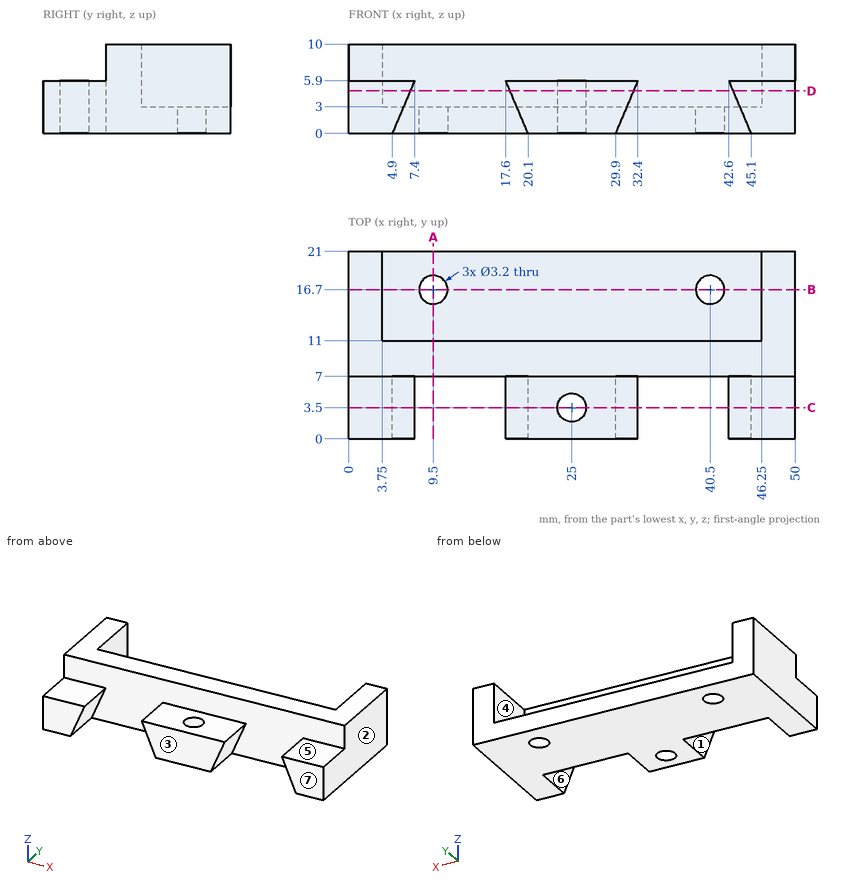
Print and shaded views of the part. All mm, measured from the part's lowest x, y and z. A direction names the side the tool comes from. Give positions to 0.01 mm unless a question says otherwise; leave off trailing zeros. Loops run counter-clockwise (first coordinate to the right, second up) from the corner with the lowest first, then second, coordinate; pieces in that order, holes last.
1) Flat gauge pins, fed straight in: pin 1 Ø2 at (x, y) = (28, 2) entering from +Z; pin 2 Ø5.5 at (x, z) = (26.5, 7) entering from +Y; pin 3 Ø2.5 at (x, y) = (40.5, 16.7) entering from +Z; pin 4 Ø1.5 at (x, y) = (41.5, 13.5) entering from +Z. Where does each tip first touch, or does it go through?
2) Wall check: line 1 (Y direction, x = 40.5, z = 0.75); line 2 (X direction, y = 17.75, z = 7.25); line 3 (X direction, y = 1.5, z = 3). Give the ranges that are in metal, low to high.
3) Pull direction X, two halves, no side cores. Call the marked faces 1, 2 and 3: +X half, -X half, draft (parallel to the pull), parting line (faces both ways), or undercut.
4) Tool access for the marked faces 4, 5, 6 and 7: list every direction of +Z, -Z, +X, -X, +Y, -Y with a clear straight run to the whole face (end or side of a thin tool).
5) Saw through at C-C (y = 3.5). Write the cut outline in (x, z), plus the area to 3 significant figures.
6) Saw through at B-B (y = 16.7). Write the cut outline in (x, z).
7) Saw through at D-D (z = 4.75). Write the cut outline in (x, y), plus the area to 3 significant figures.
8) Saw through at A-A (x = 9.5). Write the cut outline in (y, z).
Answer block:
1. pin 1: stops at z = 5.9
1. pin 2: stops at y = 11
1. pin 3: passes through
1. pin 4: stops at z = 3
2. line 1: y = 7 to 15.1, 18.3 to 21
2. line 2: x = 0 to 3.75, 46.25 to 50
2. line 3: x = 0 to 6.17, 18.83 to 31.17, 43.83 to 50
3. face 1: undercut
3. face 2: +X half
3. face 3: draft
4. face 4: +Z, +Y
4. face 5: +Z, +X, -X, -Y
4. face 6: -Z, -Y
4. face 7: +Z, -Z, +X, -X, -Y
5. outline: (0, 0) - (4.9, 0) - (7.4, 5.9) - (0, 5.9) - close; (17.6, 5.9) - (20.1, 0) - (23.4, 0) - (23.4, 5.9) - close; (26.6, 0) - (29.9, 0) - (32.4, 5.9) - (26.6, 5.9) - close; (42.6, 5.9) - (45.1, 0) - (50, 0) - (50, 5.9) - close
5. area: 126 mm2
6. outline: (0, 0) - (7.9, 0) - (7.9, 3) - (3.75, 3) - (3.75, 10) - (0, 10) - close; (11.1, 0) - (38.9, 0) - (38.9, 3) - (11.1, 3) - close; (42.1, 0) - (50, 0) - (50, 10) - (46.25, 10) - (46.25, 3) - (42.1, 3) - close
7. outline: (0, 0) - (6.91, 0) - (6.91, 7) - (18.09, 7) - (18.09, 0) - (31.91, 0) - (31.91, 7) - (43.09, 7) - (43.09, 0) - (50, 0) - (50, 21) - (46.25, 21) - (46.25, 11) - (3.75, 11) - (3.75, 21) - (0, 21) - close; hole circle Ø3.2 at (25, 3.5)
7. area: 461 mm2
8. outline: (7, 0) - (15.1, 0) - (15.1, 3) - (11, 3) - (11, 10) - (7, 10) - close; (18.3, 0) - (21, 0) - (21, 3) - (18.3, 3) - close
